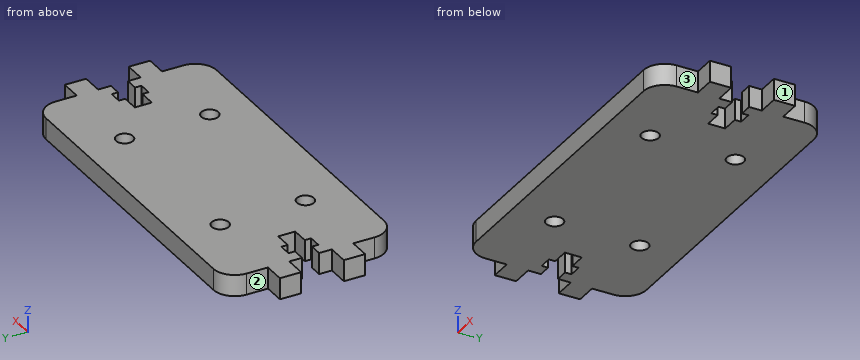
```python
from build123d import *

# Parameters (mm, degrees)
ESQUISSE1_R        = 2
BOSS_EXTRU_1_DEPTH = 5
CONG_1_R           = 5


with BuildPart() as part:
    # Esquisse1 → Boss.-Extru.1 (new body)
    with BuildSketch(Plane.XY):
        Polygon((-40, 0), (40, 0), (40, 10), (45, 10), (45, 15), (40, 15), (40, 18), (37, 18), (37, 16.5), (34, 16.5), (34, 18), (30, 18), (30, 22), (34, 22), (34, 23.5), (37, 23.5), (37, 22), (40, 22), (40, 25), (45, 25), (45, 30), (40, 30), (40, 40), (-40, 40), (-40, 30), (-45, 30), (-45, 25), (-40, 25), (-40, 22), (-37, 22), (-37, 23.5), (-34, 23.5), (-34, 22), (-30, 22), (-30, 18), (-34, 18), (-34, 16.5), (-37, 16.5), (-37, 18), (-40, 18), (-40, 15), (-45, 15), (-45, 10), (-40, 10), align=None)
        with Locations((20, 30)):
            Circle(ESQUISSE1_R, mode=Mode.SUBTRACT)
        with Locations((-20, 30)):
            Circle(ESQUISSE1_R, mode=Mode.SUBTRACT)
        with Locations((-20, 10)):
            Circle(ESQUISSE1_R, mode=Mode.SUBTRACT)
        with Locations((20, 10)):
            Circle(ESQUISSE1_R, mode=Mode.SUBTRACT)
    extrude(amount=BOSS_EXTRU_1_DEPTH)

    # Congé1
    cong_1_edges = [part.edges().sort_by_distance(p)[0] for p in [
        (40, 0, 2.5),
        (-40, 0, 2.5),
        (-40, 40, 2.5),
        (40, 40, 2.5),
    ]]
    fillet(cong_1_edges, radius=CONG_1_R)


solid = part.part
```
For this review, take the finished solid that the model builds, in its own axes (mm). Face numbers are marked on the shaded views. A direction names the side the tool comes from. Give positions to 0.01 mm unless a question says otherwise; leave off trailing zeros. Write each loop counter-clockwise with the first axis right and the second up, starting at its lowest first coordinate (ties: lowest second). Pieces come first, ordered by that corner, then holes. Notation, with made-up numbers: M -7.5,-38.5 L 47.5,-38.5 A35 cw 47.5,-4.5 Z; hole C 53.25,49.25 d10. An arc over 180 degrees is marked long. One line per item, written item: value.
1) For the marked faces 1, 2 and 3, list the 3-axis set-ups (+Z, -Z, +X, -X, +Y, -Y) from which the entire face can be reached by the end or side of a thin tool; tool diameter is ignored.
Results are:
face 1: +Z, -Z, +X, +Y, -Y
face 2: +Z, -Z, -X, +Y
face 3: +Z, -Z, +X, -Y
2) Take a section at D-D, the plane y = 20. Write out the cut boundary in (x, z).
Results are:
outline: M -30,0 L 30,0 L 30,5 L -30,5 Z
3) Take a section at B-B, the plane x = -38. Write out the cut boundary in (y, z), then the cut area to 3 significant figures.
Results are:
outline: M 1,0 L 18,0 L 18,5 L 1,5 Z; M 22,0 L 39,0 L 39,5 L 22,5 Z
area: 170 mm²
4) Take a section at A-A, the plane x = 20. Write out the cut boundary in (y, z).
Results are:
outline: M 0,0 L 8,0 L 8,5 L 0,5 Z; M 12,0 L 28,0 L 28,5 L 12,5 Z; M 32,0 L 40,0 L 40,5 L 32,5 Z
5) Take a section at C-C, the plane y = 9. Write out the cut boundary in (x, z).
Results are:
outline: M -40,0 L -21.73,0 L -21.73,5 L -40,5 Z; M -18.27,0 L 18.27,0 L 18.27,5 L -18.27,5 Z; M 21.73,0 L 40,0 L 40,5 L 21.73,5 Z
6) For P1, Ø0.8, axis at y = 23, z = 2, coming from the -X side; P2, Ø0.8, axis at y = 17, z = 3.5, coming from the +X side; P3, Ø0.9, axis at x = 38.5, z = 2, coming from the -Y side, all flat-tipped, find the tip position at first contact; note any pin that passes through.
Results are:
P1: stops at x = -40
P2: stops at x = 40
P3: stops at y = 1.04
7) For line 1 (Y direction, x = 20, z = 2.65); line 2 (X direction, y = 17, z = 0.55); line 3 (Y direction, x = 20.5, z = 4.65), list the stretches that pass through material, from the lowest coordinate up. Write a range as from..to.
Results are:
line 1: y = 0..8, 12..28, 32..40
line 2: x = -40..-37, -34..34, 37..40
line 3: y = 0..8.06, 11.94..28.06, 31.94..40
